```python
from build123d import *

# Parameters (mm, degrees)
BOSS_EXTRUDE1_DEPTH      = 100
BOSS_EXTRUDE1_DEPTH_BACK = 100
SKETCH2_W                = 135
SKETCH2_H                = 150
CUT_REVOLVE1_ANGLE       = 112.6198649
SKETCH3_R                = 20
BOSS_EXTRUDE3_DEPTH      = 30
SKETCH4_W                = 39.677312781
SKETCH4_H                = 150
CUT_EXTRUDE2_DEPTH       = 500
SKETCH7_W                = 20
SKETCH7_H                = 150


with BuildPart() as part:
    # Sketch1 → Boss-Extrude1 (new, two sides: drawn at the far end of the back side and taken through both)
    with BuildSketch(Plane(origin=(0, 0, 0), x_dir=(1, 0, 0), z_dir=(0, 1, 0)).offset(-BOSS_EXTRUDE1_DEPTH_BACK)):
        Polygon((200, 150), (300, 0), (200, -150), (-200, -150), (-200, 150), align=None)
    extrude(amount=BOSS_EXTRUDE1_DEPTH + BOSS_EXTRUDE1_DEPTH_BACK)

    # Sketch2 → Cut-Revolve1 (revolve, cut)
    with BuildSketch(Plane(origin=(207.692307692, 0, -138.461538462), x_dir=(-0.5547001962252291, 0, -0.8320502943378437), z_dir=(0.8320502943378437, 0, -0.5547001962252291))):
        with Locations((-75.066961244, 4.860296888)):
            Rectangle(SKETCH2_W, SKETCH2_H)
    revolve(axis=Axis((300, -100, 0), (0, 1, 0)), revolution_arc=CUT_REVOLVE1_ANGLE, mode=Mode.SUBTRACT)

    # Sketch3 → Boss-Extrude3 (add)
    with BuildSketch(Plane(origin=(0, 0, -150), x_dir=(-1, 0, 0), z_dir=(0, 0, -1))):
        with Locations((141.22951379, 0)):
            Circle(SKETCH3_R)
    boss_extrude3 = extrude(amount=BOSS_EXTRUDE3_DEPTH)

    # Mirror1: Boss-Extrude3 across plane
    add(boss_extrude3.mirror(Plane(origin=(0, 0, 0), x_dir=(1, 0, 0), z_dir=(0, 0, -1))))

    # Sketch4 → Cut-Extrude2 (cut)
    with BuildSketch(Plane.ZY.offset(200)):
        with Locations((-6e-09, 4.860296888)):
            Rectangle(SKETCH4_W, SKETCH4_H)
    extrude(amount=-CUT_EXTRUDE2_DEPTH, mode=Mode.SUBTRACT)

    # Sketch7 → Revolve2 (revolve)
    with BuildSketch(Plane(origin=(0, 0, 0), x_dir=(-1, 0, 0), z_dir=(0, 0, -1)), mode=Mode.PRIVATE) as revolve2_sk:
        with Locations((-290, 4.860296888)):
            Rectangle(SKETCH7_W, SKETCH7_H)
    revolve(revolve2_sk.sketch.rotate(Axis((280, 79.860296888, 0), (0, -1, 0)), 67.380135148), axis=Axis((280, 79.860296888, 0), (0, -1, 0)))


solid = part.part
```
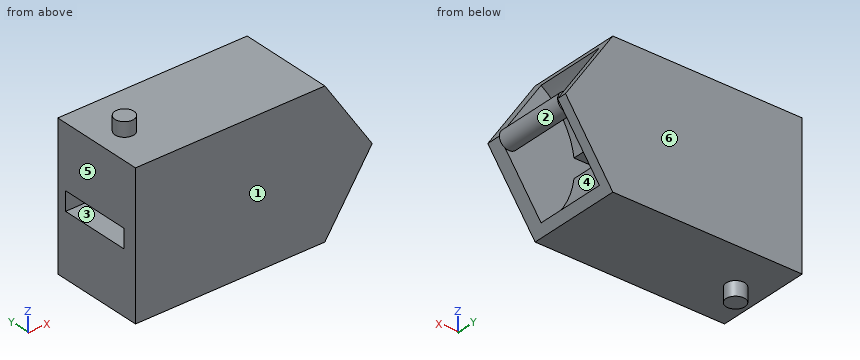
Check sheet for the modelled part. Datum: model origin and axes. Units: mm. Face numbers are marked on the shaded views. A direction names the side the tool comes from. Coordinates: 2 decimals unless noted, no trailing zeros. Write each loop counter-clockwise with the first axis right and the second up, starting at its lowest first coordinate (ties: lowest second). Pieces come first, ordered by that corner, then holes. Notation, with made-up numbers: M -36.5,-11.5 L -9.5,-11.5 A21 cw -9.5,11.5 Z; hole C 69.5,-17.75 d4. An arc over 180 degrees is marked long. Write item = value, one per line. Start each with the question number.
1. Thickness scan on probe 1 along Z at (x, y) = (-21, 2.5); probe 2 along Z at (x, y) = (-157, -9.5); probe 3 along Y at (x, z) = (62, -17). Record the ranges inside material, lowest first.
2. Sectioned sample at B-B (x = 280). Record the cut outline in (y, z).
3. Sectioned sample at A-A (y = 0). Record the cut outline in (x, z), then the cut area to 3 significant figures.
4. Go/stop test with flat-tipped pins: pin 1 (3 mm diameter, centred on x = 49.5, y = -39.5, fed in from -Z); pin 2 (13.5 mm diameter, centred on x = 295.5, z = 8.5, fed in from -Y); pin 3 (2 mm diameter, centred on x = -141, y = 55.5, fed in from +Z); pin 4 (1.5 mm diameter, centred on y = 73.5, z = 107, fed in from +X). Record where each tip stops, or that it passes through.
5. Mould release check, pull along Y, two halves, no side actions. Record for the marked faces 4, 5 and 6: pulls with the +Y half, pulls with the -Y half, needs draft (parallel to the pull), parting line crosses it, or undercut.
6. Sectioned sample at D-D (z = -12.5). Record the cut outline in (x, y), then the cut area to 3 significant figures.
7. Sectioned sample at C-C (x = 37). Record the cut outline in (y, z).
8. Tool access check on the marked faces 1, 2 and 3. Record the directions out of +Z, -Z, +X, -X, +Y, -Y that give a thin tool (end or side, any length) a straight path to the whole face; none if there is none.
The answers:
q1.probe_1 = -150 to -19.84, 19.84 to 150
q1.probe_2 = -180 to -19.84, 19.84 to 180
q1.probe_3 = -100 to -70.14, 79.86 to 100
q2.outline = M -100,-30 L -70.14,-30 L -70.14,-20 L 79.86,-20 L 79.86,-30 L 100,-30 L 100,30 L 79.86,30 L 79.86,20 L -70.14,20 L -70.14,30 L -100,30 Z
q3.outline = M -200,-150 L -161.23,-150 L -161.23,-180 L -121.23,-180 L -121.23,-150 L 200,-150 L 211.89,-132.17 A158.84 cw 142.4,-19.84 L -200,-19.84 Z; M -200,19.84 L 142.4,19.84 A158.84 cw 211.89,132.17 L 200,150 L -121.23,150 L -121.23,180 L -161.23,180 L -161.23,150 L -200,150 Z; C 280,0 d40
q3.area = 100,000 mm²
q4.pin_1 = -150
q4.pin_2 = -100
q4.pin_3 = 150
q4.pin_4 = 183.29
q5.face_4 = undercut
q5.face_5 = needs draft
q5.face_6 = pulls with the +Y half
q6.outline = M -200,-100 L 291.67,-100 L 291.67,-70.14 L 295.61,-70.14 L 295.61,79.86 L 291.67,79.86 L 291.67,100 L -200,100 L -200,79.86 L 264.39,79.86 L 264.39,-70.14 L -200,-70.14 Z
q6.area = 29,300 mm²
q7.outline = M -100,-150 L 100,-150 L 100,150 L -100,150 Z; hole M -70.14,-19.84 L 79.86,-19.84 L 79.86,19.84 L -70.14,19.84 Z
q8.face_1 = +Z, -Z, +X, -X, -Y
q8.face_2 = none
q8.face_3 = -X
